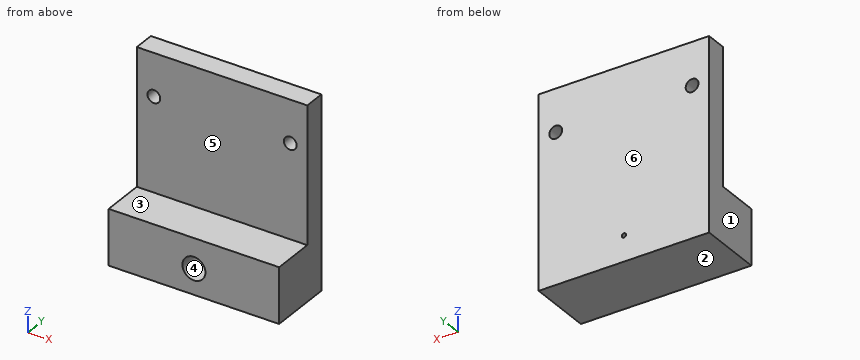
from build123d import *

# Parameters (mm, degrees)
F0_W      = 40
F0_H      = 45
F1_DEPTH  = 15
F2_R      = 1.5
F3_DEPTH  = 25
F7_R      = 2.7
F8_DEPTH  = 10
F9_W      = 40
F9_H      = 32
F10_DEPTH = 10
F11_R     = 0.5
F12_DEPTH = 15


with BuildPart() as f1:
    # F0 (on Front) → F1 (new body)
    with BuildSketch(Plane.XZ):
        Rectangle(F0_W, F0_H)
    extrude(amount=F1_DEPTH)

    # F2 (on face) → F3 (cut)
    with BuildSketch(Plane.XZ.offset(15)):
        with Locations((16, 12.5)):
            Circle(F2_R)
        with Locations((-16, 12.5)):
            Circle(F2_R)
    extrude(amount=-F3_DEPTH, mode=Mode.SUBTRACT)

    # F7 (on face) → F8 (cut)
    with BuildSketch(Plane.XZ.offset(15)):
        with Locations((0, -16.5)):
            Circle(F7_R)
    extrude(amount=-F8_DEPTH, mode=Mode.SUBTRACT)

    # F9 (on face) → F10 (cut)
    with BuildSketch(Plane.XZ.offset(15)):
        with Locations((0, 6.5)):
            Rectangle(F9_W, F9_H)
    extrude(amount=-F10_DEPTH, mode=Mode.SUBTRACT)

    # F11 (on face) → F12 (cut)
    with BuildSketch(Plane.XZ.offset(15)):
        with Locations((0, -16.5)):
            Circle(F11_R)
    extrude(amount=-F12_DEPTH, mode=Mode.SUBTRACT)


solid = f1.part
Read the model definition and answer for the solid it produces. Units are mm, in the model's axes. Face numbers are marked on the shaded views. A direction names the side the tool comes from. Give positions to 0.01 mm unless a question says otherwise; leave off trailing zeros. Write each loop counter-clockwise with the first axis right and the second up, starting at its lowest first coordinate (ties: lowest second). Pieces come first, ordered by that corner, then holes. Notation, with made-up numbers: (69.25, 56) - (82.25, 56) arc R28 cw to (82.25, 92) - close; hole circle Ø11 at (18.25, 73). An arc over 180 degrees is marked (long way). Use CSV: the item, a comma, the result in double quotes. Start each with the question number.
(1) For the marked faces 5 and 6, determine the directions among +Z, -Z, +X, -X, +Y, -Y from which every point of the face is accessible in a straight line to the end or side of a thin tool.
(2) Find section D-D (x = 0). Give the vertices of the cut face in (y, z), plus the area to 3 significant figures.
(3) Find section B-B (x = -16). Give the vertices of the cut face in (y, z).
(4) Determine the mould class of the marked faces 1, 2, 3 and 4 for opening direction Z: +Z half, -Z half, draft (parallel to the pull), parting line (faces both ways), or undercut.
(5) Given P1, Ø1.5, axis at x = 12, y = -7.5, coming from the +Z side; P2, Ø5, axis at x = 16, z = 12.5, coming from the -Y side, each flat-ended and moving along its own axis, determine where each tip first touches the part or whether it passes through.
(6) Consider line 1 along Z through (x, y) = (-16, -1.95); line 2 along Z through (x, y) = (15, -12); line 3 along Y through (x, z) = (0.5, -8). Determine where each line is inside the solid, lowest interval first.
(7) Find section A-A (z = 12.5). Give the vertices of the cut face in (x, y).
(8) Find section C-C (y = -7). Give the vertices of the cut face in (x, z), plus the area to 3 significant figures.
Findings below:
1,face 5,"+Z, +X, -X, -Y"
1,face 6,"+Z, -Z, +X, -X, +Y"
2,outline,"(-15, -22.5) - (0, -22.5) - (0, -17) - (-5, -17) - (-5, -19.2) - (-15, -19.2) - close; (-15, -13.8) - (-5, -13.8) - (-5, -16) - (0, -16) - (0, 22.5) - (-5, 22.5) - (-5, -9.5) - (-15, -9.5) - close"
2,area,"296 mm2"
3,outline,"(-15, -22.5) - (0, -22.5) - (0, 11) - (-5, 11) - (-5, -9.5) - (-15, -9.5) - close; (-5, 14) - (0, 14) - (0, 22.5) - (-5, 22.5) - close"
4,face 1,"draft"
4,face 2,"-Z half"
4,face 3,"+Z half"
4,face 4,"undercut"
5,P1,"z = -9.5"
5,P2,"y = -5"
6,line 1,"-22.5 to 11, 14 to 22.5"
6,line 2,"-22.5 to -9.5"
6,line 3,"-5 to 0"
7,outline,"(-20, -5) - (-17.5, -5) - (-17.5, 0) - (-20, 0) - close; (-14.5, -5) - (14.5, -5) - (14.5, 0) - (-14.5, 0) - close; (17.5, -5) - (20, -5) - (20, 0) - (17.5, 0) - close"
8,outline,"(-20, -22.5) - (20, -22.5) - (20, -9.5) - (-20, -9.5) - close; hole circle Ø5.4 at (0, -16.5)"
8,area,"497 mm2"
